from build123d import *

# Parameters (mm, degrees)
SKETCH1_R           = 9.525
BOSS_EXTRUDE1_DEPTH = 50.8
SKETCH2_R           = 2.4765
CUT_EXTRUDE1_DEPTH  = 20.05


with BuildPart() as part:
    # Sketch1 → Boss-Extrude1 (new body)
    with BuildSketch(Plane(origin=(0, 0, 0), x_dir=(1, 0, 0), z_dir=(0, 1, 0))):
        Circle(SKETCH1_R)
        with BuildLine():
            Line((2.439590334, 2.032), (2.439590334, -2.032))
            ThreePointArc((2.439590334, -2.032), (-3.175, 0), (2.439590334, 2.032))
        make_face(mode=Mode.SUBTRACT)
    extrude(amount=BOSS_EXTRUDE1_DEPTH)

    # Sketch2 → Cut-Extrude1 (cut, through all)
    with BuildSketch(Plane.XY.offset(9.525)):
        with Locations((0, 9.525)):
            Circle(SKETCH2_R)
        with Locations((0, 22.225)):
            Circle(SKETCH2_R)
    extrude(amount=-CUT_EXTRUDE1_DEPTH, mode=Mode.SUBTRACT)


solid = part.part
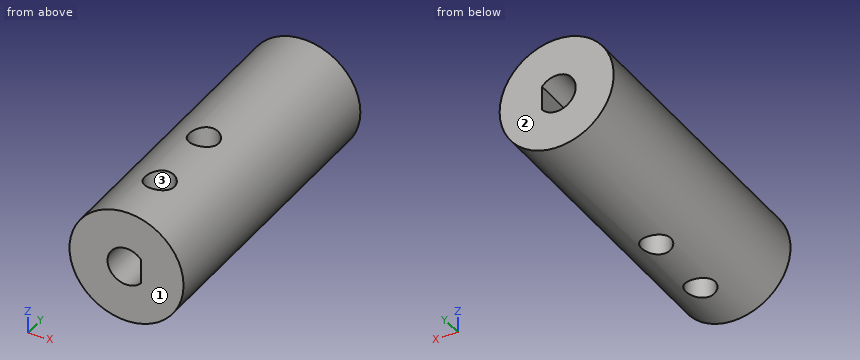
Source: CAD feature listing. Evaluate the final solid. Frame: model axes, mm. Face numbers are marked on the shaded views. Round coordinates to 2 decimals unless told otherwise and drop trailing zeros. Order: outer loops, then holes, each group sorted by start corner. A loop starts at its lowest first (then second) coordinate and runs counter-clockwise, first axis right, second up. Notation, with made-up numbers: (44, 35.25) - (55, 35.25) arc R20 ccw to (55, 52.25) - close; hole circle Ø8 at (-39, 70.25). An arc over 180 degrees is marked (long way). Use a Markdown table: item, result. Add a question column.
1. First-contact query: pin 1 (10 mm diameter, centred on y = 26.5, z = 6.5, fed in from -X); pin 2 (8 mm diameter, centred on y = 38.5, z = 6.5, fed in from +X); pin 3 (4 mm diameter, centred on y = 6, z = 6.5, fed in from -X) (3 decimals). Flat tips, straight axial feed; report the tip coordinate or a pass-through.
2. Section query C-C (y = 11.5). Return the cut outline in (x, z) (3 decimals).
3. Line query: probe 1 along Z at (x, y) = (0, 29.5) (3 decimals); probe 2 along Y at (x, z) = (-2.25, 7); probe 3 along X at (y, z) = (11.5, 0) (3 decimals). Output: solid intervals per line, ascending.
4. Section query D-D (z = -7.5). Return the cut outline in (x, y) (1 decimal), then the cut area to 3 significant figures.
5. Section query B-B (z = 0). Return the cut outline in (x, y) (1 decimal), then the cut area to 3 significant figures.
6. Section query A-A (x = 0). Return the cut outline in (y, z) (1 decimal), then the cut area to 3 significant figures.
7. Mould query, pull axis Y, two halves, no side actions, for the marked faces 1, 2 and 3. Classes: +Y half, -Y half, draft (parallel to the pull), parting line (faces both ways), or undercut.
Derived:
| question | item | result |
|---|---|---|
| 1 | pin 1 | x = -9.41 |
| 1 | pin 2 | x = 9.19 |
| 1 | pin 3 | x = -8.395 |
| 2 | outline | (-1.494, -9.407) - (-1.494, -2.801) arc R3.175 cw to (-1.494, 2.801) - (-1.494, 9.407) arc R9.525 ccw to start; (1.494, -9.407) arc R9.525 ccw to (1.494, 9.407) - (1.494, 2.801) arc R3.175 cw to (2.44, 2.032) - (2.44, -2.032) arc R3.175 cw to (1.494, -2.801) - close |
| 3 | probe 1 | -9.525 to -3.175, 3.175 to 9.525 |
| 3 | probe 2 | 0 to 8.49, 10.56 to 21.19, 23.26 to 50.8 |
| 3 | probe 3 | -9.525 to -3.175, 2.44 to 9.525 |
| 4 | outline | (-5.9, 0) - (5.9, 0) - (5.9, 50.8) - (-5.9, 50.8) - close; hole circle Ø5 at (0, 9.5); hole circle Ø5 at (0, 22.2) |
| 4 | area | 558 mm2 |
| 5 | outline | (-9.5, 0) - (-3.2, 0) - (-3.2, 50.8) - (-9.5, 50.8) - close; (2.4, 0) - (9.5, 0) - (9.5, 50.8) - (2.4, 50.8) - (2.4, 22.7) arc R2.5 cw to (2.4, 21.8) - (2.4, 10) arc R2.5 cw to (2.4, 9.1) - close |
| 5 | area | 682 mm2 |
| 6 | outline | (0, -9.5) - (7, -9.5) - (7, -3.2) - (0, -3.2) - close; (0, 3.2) - (7, 3.2) - (7, 9.5) - (0, 9.5) - close; (12, -9.5) - (19.7, -9.5) - (19.7, -3.2) - (12, -3.2) - close; (12, 3.2) - (19.7, 3.2) - (19.7, 9.5) - (12, 9.5) - close; (24.7, -9.5) - (50.8, -9.5) - (50.8, -3.2) - (24.7, -3.2) - close; (24.7, 3.2) - (50.8, 3.2) - (50.8, 9.5) - (24.7, 9.5) - close |
| 6 | area | 519 mm2 |
| 7 | face 1 | -Y half |
| 7 | face 2 | +Y half |
| 7 | face 3 | undercut |
